Verification items for the finished model (mm, model axes). A direction names the side the tool comes from. Give positions to 0.01 mm unless a question says otherwise; leave off trailing zeros. Loops run counter-clockwise (first coordinate to the right, second up) from the corner with the lowest first, then second, coordinate; pieces in that order, holes last. Notation, with made-up numbers: (-1, 7) - (40, 7) arc R34 cw to (40, 45) - close; hole circle Ø6 at (35, 1). An arc over 180 degrees is marked (long way). One line per question, with ' | ' between items. Start each with the question number.
1. Tool access check on faces 4 (the face through (58.996, 27.31, 8.254)), 5 (the face through (-65.865, 22.794, 1.504)). Record the directions out of +Z, -Z, +X, -X, +Y, -Y that give a thin tool (end or side, any length) a straight path to the whole face; none if there is none.
2. Mould release check, pull along X, two halves, no side actions. Record for faces 1 (the face through (-65.865, -11.122, 6.774)), 2 (the face through (66.205, -11.2, 6.774)), 3 (the face through (56, 22, 8)): +X half, -X half, draft (parallel to the pull), parting line (faces both ways), or undercut.
3. Section check C-C, the plane x = 58. Enter the section's corners in (y, z).
4. Section check B-B, the plane z = 2.5. Enter the section's corners in (x, y).
5. Thickness scan on line 1 along Z through (x, y) = (27, -8); line 2 along X through (y, z) = (41, 1.75); line 3 along X through (y, z) = (21, 3.75). Record the ranges inside material, lowest first. Write a range as from..to.
6. Depth check by flat-ended pin: pin 1 Ø3 at (x, z) = (-26, 3) entering from +Y. Enter the tip coordinate at first touch or a pass-through.
7. Section check A-A, the plane x = -36.5. Enter the section's corners in (y, z), then the cut area to 3 significant figures.
from build123d import *

# Parameters (mm, degrees)
F0_W     = 135
F0_H     = 70
F1_DEPTH = 8.5
F2_R     = 5
F3_R     = 5
F4_R     = 5.85347
F5_DEPTH = 0.5


with BuildPart() as f1:
    # F0 (on Top) → F1 (new body)
    with BuildSketch(Plane.XY):
        with Locations((0.209052, 22.374493)):
            Rectangle(F0_W, F0_H)
    extrude(amount=F1_DEPTH)

    # F2
    f2_edges = [f1.edges().sort_by_distance(p)[0] for p in [
        (67.709052, -12.625507, 4.25),
        (67.709052, 57.374493, 4.25),
        (-67.290948, -12.625507, 4.25),
        (-67.290948, 57.374493, 4.25),
    ]]
    fillet(f2_edges, radius=F2_R)

    # F3
    f3_edges = [f1.edges().sort_by_distance(p)[0] for p in [
        (-67.290948, 22.374493, 0),
    ]]
    fillet(f3_edges, radius=F3_R)

    # F4 (on face) → F5 (cut)
    with BuildSketch(Plane.XY.offset(8.5)):
        with Locations((55.848766, 22.374493)):
            Circle(F4_R)
    extrude(amount=-F5_DEPTH, mode=Mode.SUBTRACT)


solid = f1.part
Results list:
1) face 4: +Z | face 5: -Z, -X, +Y, -Y
2) face 1: -X half | face 2: +X half | face 3: undercut
3) outline: (-12.63, 5) arc R5 ccw to (-7.63, 0) - (52.37, 0) arc R5 ccw to (57.37, 5) - (57.37, 8.5) - (27.82, 8.5) - (27.82, 8) - (16.93, 8) - (16.93, 8.5) - (-12.63, 8.5) - close
4) outline: (-66.62, -7.63) arc R4.33 ccw to (-62.29, -11.96) - (62.71, -11.96) arc R4.33 ccw to (67.04, -7.63) - (67.04, 52.37) arc R4.33 ccw to (62.71, 56.7) - (-62.29, 56.7) arc R4.33 ccw to (-66.62, 52.37) - close
5) line 1: 0.01..8.5 | line 2: -66.09..66.51 | line 3: -67.13..67.55
6) pin 1: y = 57.35
7) outline: (-12.63, 5) arc R5 ccw to (-7.63, 0) - (52.37, 0) arc R5 ccw to (57.37, 5) - (57.37, 8.5) - (-12.63, 8.5) - close | area: 584 mm²
